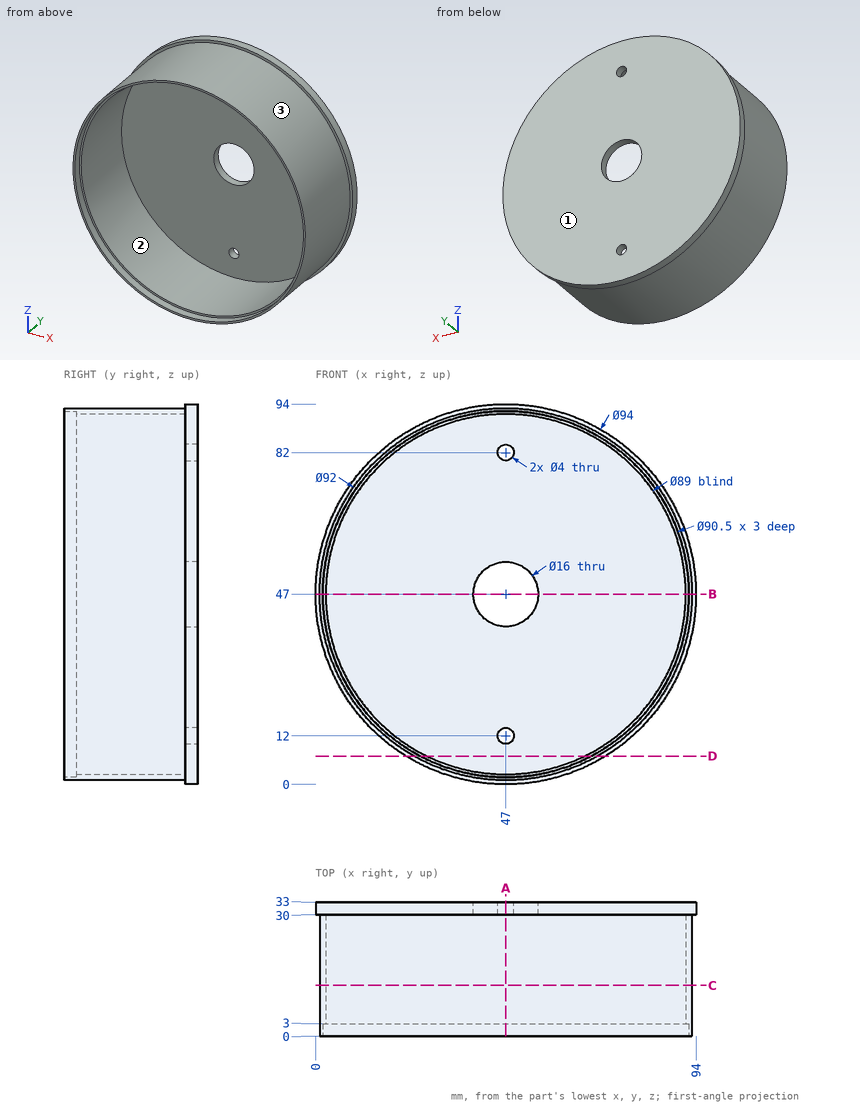
Geometry check sheet. Reference: drawing and pictorial views, mm from the part's lowest x, y, z. Round coordinates to 2 decimals unless told otherwise and drop trailing zeros. Loops run counter-clockwise (first coordinate to the right, second up) from the corner with the lowest first, then second, coordinate; pieces in that order, holes last. Notation, with made-up numbers: (-4, 35.5) - (43, 35.5) arc R23 ccw to (43, 46.5) - close; hole circle Ø10 at (30, 5.5). An arc over 180 degrees is marked (long way). Answer as CSV lines item,"result".
(1) Material ranges on line 1 along X through (y, z) = (16, 47); line 2 along X through (y, z) = (1.6, 47); line 3 along Z through (x, y) = (83.5, 14), recorded low to high.
Output values:
line 1,"x = 1 to 2.5, 91.5 to 93"
line 2,"x = 1 to 1.75, 92.25 to 93"
line 3,"z = 19 to 21.54, 72.46 to 75"
(2) Release check for a two-part mould opening along Z. For the marked faces 1, 2 and 3 record: released by +Z, released by -Z, zero draft, split by the parting line, or undercut.
Output values:
face 1,"zero draft"
face 2,"undercut"
face 3,"split by the parting line"
(3) Cross-section at D-D, the plane z = 7. Enter the section's corners in (x, y).
Output values:
outline,"(22.32, 30) - (24.28, 30) - (24.28, 0) - (25.84, 0) - (25.84, 3) - (27.5, 3) - (27.5, 30) - (66.5, 30) - (66.5, 3) - (68.16, 3) - (68.16, 0) - (69.72, 0) - (69.72, 30) - (71.68, 30) - (71.68, 33) - (22.32, 33) - close"
(4) Cross-section at C-C, the plane y = 12.5. Enter the section's corners in (x, z).
Output values:
outline,"circle Ø92 at (47, 47); hole circle Ø89 at (47, 47)"
(5) Cross-section at A-A, the plane x = 47. Enter the section's corners in (y, z).
Output values:
outline,"(0, 1) - (30, 1) - (30, 0) - (33, 0) - (33, 10) - (30, 10) - (30, 2.5) - (3, 2.5) - (3, 1.75) - (0, 1.75) - close; (0, 92.25) - (3, 92.25) - (3, 91.5) - (30, 91.5) - (30, 84) - (33, 84) - (33, 94) - (30, 94) - (30, 93) - (0, 93) - close; (30, 14) - (33, 14) - (33, 39) - (30, 39) - close; (30, 55) - (33, 55) - (33, 80) - (30, 80) - close"
(6) Depth check by flat-ended pin: pin 1 Ø1.5 at (x, y) = (59, 14.5) entering from +Z; pin 2 Ø5 at (x, y) = (20.5, 10) entering from +Z; pin 3 Ø1 at (x, y) = (36.5, 7) entering from -Z. Enter the tip coordinate at first touch or a pass-through.
Output values:
pin 1,"stops at z = 91.6"
pin 2,"stops at z = 86.24"
pin 3,"stops at z = 2.1"
(7) Cross-section at B-B, the plane z = 47. Enter the section's corners in (x, y), and give its area (4 significant figures).
Output values:
outline,"(0, 30) - (1, 30) - (1, 0) - (1.75, 0) - (1.75, 3) - (2.5, 3) - (2.5, 30) - (39, 30) - (39, 33) - (0, 33) - close; (55, 30) - (91.5, 30) - (91.5, 3) - (92.25, 3) - (92.25, 0) - (93, 0) - (93, 30) - (94, 30) - (94, 33) - (55, 33) - close"
area,"319.5 mm²"
